Input: dimensioned drawing with shaded views. Units: mm. Origin: part minimum x, y, z. Coordinates: 2 decimals unless noted, no trailing zeros. Loops run counter-clockwise (first coordinate to the right, second up) from the corner with the lowest first, then second, coordinate; pieces in that order, holes last.
(1) Section B-B, the plane x = 9.5. Return loops of the section in (y, z).
(2) Line query: L1, parallel to X at y = 1, z = 8.75; L2, parallel to X at y = 3.75, z = 8; L3, parallel to Z at x = 10, y = 3. Output: solid intervals per line, ascending.
(3) Mould query, pull axis Z, two halves, no side actions, for the marked faces 1, 2, 3 and 4. Classes: released by +Z, released by -Z, zero draft, split by the parting line, or undercut.
(4) Section A-A, the plane z = 9. Return loops of the section in (x, y).
(5) Section C-C, the plane y = 4.5. Return loops of the section in (x, z).
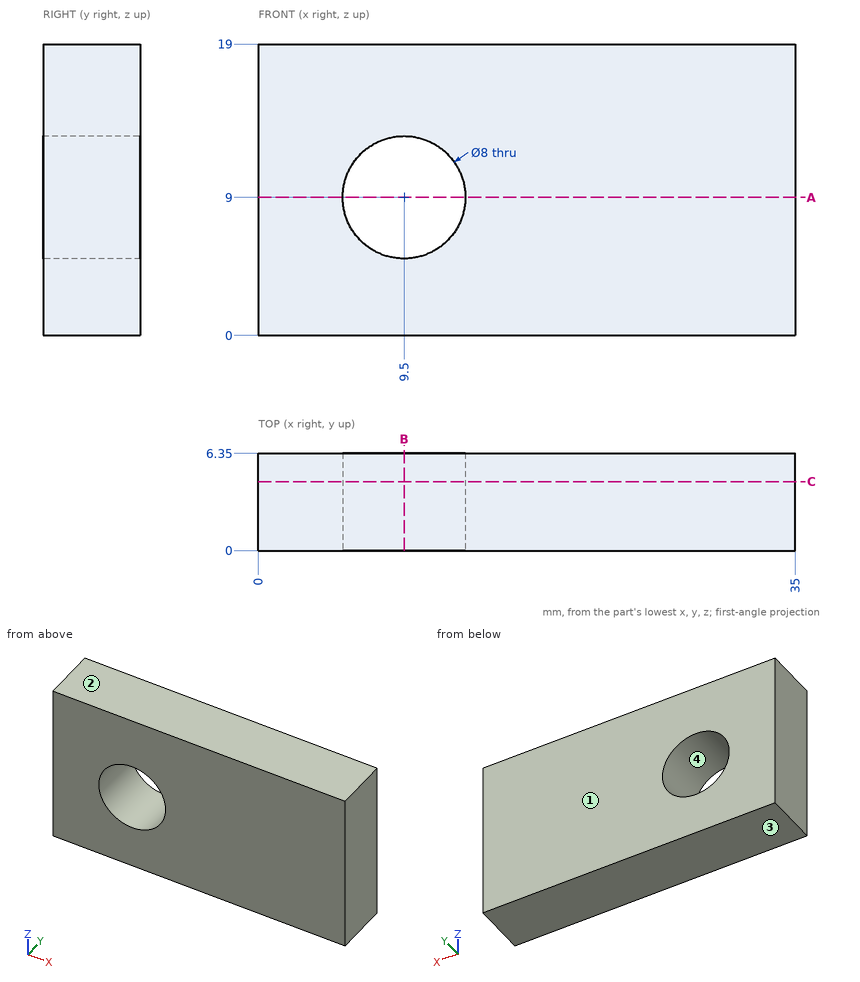
Report:
1. outline: (0, 0) - (6.35, 0) - (6.35, 5) - (0, 5) - close; (0, 13) - (6.35, 13) - (6.35, 19) - (0, 19) - close
2. L1: x = 0 to 5.51, 13.49 to 35
2. L2: x = 0 to 5.63, 13.37 to 35
2. L3: z = 0 to 5.03, 12.97 to 19
3. face 1: zero draft
3. face 2: released by +Z
3. face 3: released by -Z
3. face 4: undercut
4. outline: (0, 0) - (5.5, 0) - (5.5, 6.35) - (0, 6.35) - close; (13.5, 0) - (35, 0) - (35, 6.35) - (13.5, 6.35) - close
5. outline: (0, 0) - (35, 0) - (35, 19) - (0, 19) - close; hole circle Ø8 at (9.5, 9)
